Input: part model. Units: mm. Frame: model coordinates. Face numbers are marked on the shaded views. Give positions to 0.01 mm unless a question says otherwise; leave off trailing zeros. Loops run counter-clockwise (first coordinate to the right, second up) from the corner with the lowest first, then second, coordinate; pieces in that order, holes last. Notation, with made-up numbers: M -13,41 L 35,41 A24 cw 35,75 Z; hole C 13.25,5.25 d4. An arc over 180 degrees is marked long. Return JSON: item names as keys, results as strings. Group by question number.
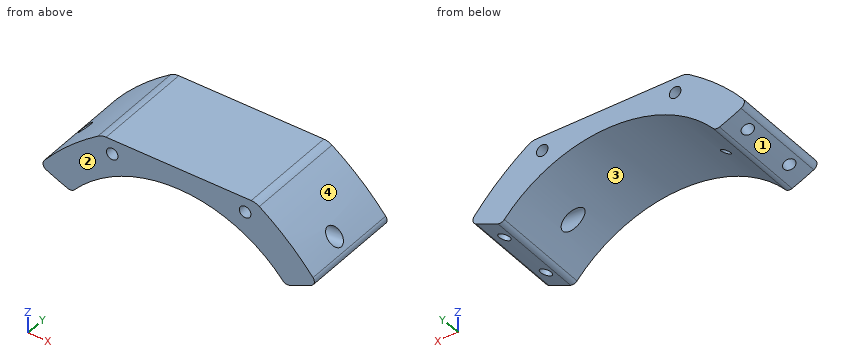
Autodesk Inventor part; units mm, degrees
ref_plane "РабПлоскость9" through (-46.2409, 0, 45.7515) normal (0.4007, 0, 0.9162) x (0, -1, 0)
ref_plane "РабПлоскость12" through (46.4848, 0, 49.7456) normal (-0.9962, 0, -0.0872) x (0, -1, 0)
ref_plane "РабПлоскость13" through (-46.505, 0, 49.7461) normal (-0.998, 0, 0.0634) x (0, 1, 0)
sketch "Эскиз1" plane through (0, 0, 0) normal (0, 1, 0) x (-1, 0, 0)
  line L0 (-25.0999, 67.4751) -> (25.1202, 67.4751)
  arc A0 (37.0101, 42.8778) -> (-36.9899, 42.8778) centre (0.0101, 12.3) ccw
  arc A1 (36.6633, -21.4663) -> (-36.0003, -21.4663) centre (0.3315, -28.4663) ccw
  line L1 (36.6633, -21.4663) -> (-36.0003, -21.4663)
  circle A2 centre (23.0101, 62.4751) radius 2
  arc A3 (37.0101, 42.8778) -> (48.0857, 47.7907) centre (0.4498, 140.2397) ccw
  circle A4 centre (-22.9899, 62.4751) radius 2
  arc A5 (-48.0655, 47.7901) -> (-36.9899, 42.8778) centre (-0.4338, 140.2412) ccw
  arc A6 (-27.9123, 66.6091) -> (-48.0655, 47.7901) centre (22.7111, -7.8037) ccw
  arc A7 (48.0857, 47.7907) -> (27.9326, 66.6092) centre (-22.6902, -7.8041) ccw
  arc A8 (27.9326, 66.6092) -> (25.1202, 67.4751) centre (25.1202, 62.4751) ccw
  arc A9 (-25.0999, 67.4751) -> (-27.9123, 66.6091) centre (-25.0999, 62.4751) ccw
  line L2 (37.0101, 42.8778) -> (-36.9899, 42.8778)
  point P0 (0, 0)
  point P1 (0, 0)
  point P2 (-26.6154, 67.4751)
  point P3 (0.0101, 60.3)
  point P4 (0.0102, 67.4751)
  point P5 (0, 0)
  point P6 (26.6357, 67.4751)
  point P7 (-26.5712, 67.2537)
  point P8 (26.5916, 67.2537)
  dimension "d0" = 72.6636
  dimension "d1" = 37
  dimension "d2" = 11.0756
  dimension "d3" = 7.1751
  dimension "d4" = 5
  dimension "d5" = 5
  dimension "d6" = 90
  dimension "d7" = 90
  dimension "d8" = 5
  dimension "d95" = 23
  dimension "d96" = 23
  dimension "d97" = 48
  dimension "d98" = 11.0756
  dimension "d105" = 74
  dimension "d107" = 4
  dimension "d108" = 4
extrude "Выдавливание1" add sketch "Эскиз1" along normal blind 35 contours L0 A8 A7 A3 A0 A5 A6 A9
fillet "Сопряжение2" radius 2 4 edges at (48.0655, 17.5, 47.7901) (36.9899, 17.5, 42.8778) (-37.0101, 17.5, 42.8778) (-48.0857, 17.5, 47.7907)
ref_plane "РабПлоскость4" through (38.3242, 0, 43.3892) normal (0.3643, 0, -0.9313) x (0, 1, 0)
sketch "Эскиз9" plane through (38.3242, 0, 43.3892) normal (0.3643, 0, -0.9313) x (0, 1, 0)
  circle A0 centre (27.5, 3.3848) radius 2
  circle A1 centre (7.5, 3.3848) radius 2
  line L0 (35, 0) -> (35, 8.1748)
  line L1 (0, 8.1748) -> (35, 8.1748)
  point P0 (0, -51.4982)
  dimension "d49" = 4
  dimension "d50" = 4
  dimension "d51" = 20
  dimension "d52" = 7.5
  dimension "d53" = 4.79
  dimension "d54" = 4.79
extrude "Выдавливание6" cut sketch "Эскиз9" against normal blind 10
ref_plane "РабПлоскость9" through (-46.2409, 0, 45.7515) normal (0.4007, 0, 0.9162) x (0, -1, 0)
ref_plane "РабПлоскость8" through (-45.8402, 0, 46.6678) normal (0.4007, 0, 0.9162) x (0, -1, 0)
sketch "Эскиз12" plane through (-46.2409, 0, 45.7515) normal (0.4007, 0, 0.9162) x (0, -1, 0)
  circle A0 centre (-27.5, 3.3914) radius 2
  circle A1 centre (-7.5, 3.3914) radius 2
  line L0 (0, 8.1814) -> (-35, 8.1814)
  line L1 (-35, 8.1814) -> (-35, 0)
  point P0 (0, 60.6995)
  dimension "d66" = 4
  dimension "d67" = 4
  dimension "d68" = 20
  dimension "d69" = 4.79
  dimension "d70" = 4.79
  dimension "d71" = 7.5
extrude "Выдавливание8" cut sketch "Эскиз12" along normal blind 10
ref_plane "РабПлоскость12" through (46.4848, 0, 49.7456) normal (-0.9962, 0, -0.0872) x (0, -1, 0)
sketch "Эскиз14" plane through (46.4848, 0, 49.7456) normal (-0.9962, 0, -0.0872) x (0, -1, 0)
  circle A0 centre (-15, 4) radius 2.75
  line L0 (0, 18.418) -> (0, 0)
  line L1 (-35, 0) -> (0, 0)
  point P0 (0, -45.5049)
  dimension "d78" = 5.5
  dimension "d79" = 15
  dimension "d80" = 4
extrude "Выдавливание9" cut sketch "Эскиз14" along normal blind 43.25
ref_plane "РабПлоскость13" through (-46.505, 0, 49.7461) normal (-0.998, 0, 0.0634) x (0, 1, 0)
sketch "Эскиз16" plane through (-46.505, 0, 49.7461) normal (-0.998, 0, 0.0634) x (0, 1, 0)
  circle A0 centre (15, -4) radius 2.25
  line L0 (0, -18.0062) -> (0, 0)
  line L1 (0, 0) -> (35, 0)
  point P0 (0, 46.6988)
  dimension "d85" = 4.5
  dimension "d86" = 15
  dimension "d87" = 4
extrude "Выдавливание10" cut sketch "Эскиз16" against normal blind 15.5
sketch "Эскиз17" plane through (-46.505, 0, 49.7461) normal (-0.998, 0, 0.0634) x (0, 1, 0)
  circle A0 centre (15, -4) radius 1.25
  line L0 (0, -18.0062) -> (0, 0)
  line L1 (0, 0) -> (35, 0)
  point P0 (0, 46.6988)
  dimension "d90" = 2.5
  dimension "d91" = 15
  dimension "d92" = 4
extrude "Выдавливание11" cut sketch "Эскиз17" against normal blind 31.25
properties part number "dribler_ball"
Item 1: Section C-C, the plane y = 23.5. Give the number of separate pieces and of enclosed holes in the cut face, then the cut area to 3 significant figures.
Item 2: First-contact query: pin 1 Ø2.5 at (x, z) = (-23.01, 62.48) entering from +Y; pin 2 Ø6 at (y, z) = (4.5, 61.5) entering from -X; pin 3 Ø5 at (y, z) = (30, 54) entering from -X; pin 4 Ø3 at (x, y) = (31.5, 20.5) entering from -Z. Flat tips, straight axial feed; report the tip coordinate or a pass-through.
Item 3: Section D-D, the plane x = -11. Return loops of the section in (y, z), then the cut area to 3 significant figures.
Item 4: Pull-direction query (X, two-part tool) for the marked faces 1, 2, 3 and 4; classes: pulls with the +X half, pulls with the -X half, needs draft (parallel to the pull), parting line crosses it, or undercut.
Item 5: Material intervals for line 1 (X direction, y = 29.5, z = 61); line 2 (X direction, y = 5, z = 61.75); line 3 (X direction, y = 21.5, z = 48.25), sorted ascending. Write a range as from..to.
Item 6: Section A-A, the plane z = 63.5. Return loops of the section in (x, y).
Item 7: Section B-B, the plane x = 20. Return loops of the section in (y, z), then the cut area to 3 significant figures.
Answer below:
{
 "1": {"separate pieces": "1", "enclosed holes": "2", "area": "1,010 mm^2"},
 "2": {"pin 1": "through", "pin 2": "x = -38.17", "pin 3": "x = -45.01", "pin 4": "z = 47.15"},
 "3": {"outline": "M 0,59.02 L 35,59.02 L 35,67.48 L 0,67.48 Z", "area": "296 mm^2"},
 "4": {"face 1": "pulls with the -X half", "face 2": "needs draft", "face 3": "undercut", "face 4": "pulls with the +X half"},
 "5": {"line 1": "-35.33..-24.36, -21.66..21.64, 24.34..35.31", "line 2": "-34.43..-24.87, -21.15..21.13, 24.85..34.41", "line 3": "-46.96..-31.82, 31.8..46.94"},
 "6": {"outline": "M -32.23,0 L -24.73,0 L -24.73,35 L -32.23,35 Z; M -21.29,0 L 21.27,0 L 21.27,35 L -21.29,35 Z; M 24.71,0 L 32.2,0 L 32.2,35 L 24.71,35 Z"},
 "7": {"outline": "M 0,55.93 L 35,55.93 L 35,67.48 L 0,67.48 Z", "area": "404 mm^2"}
}
